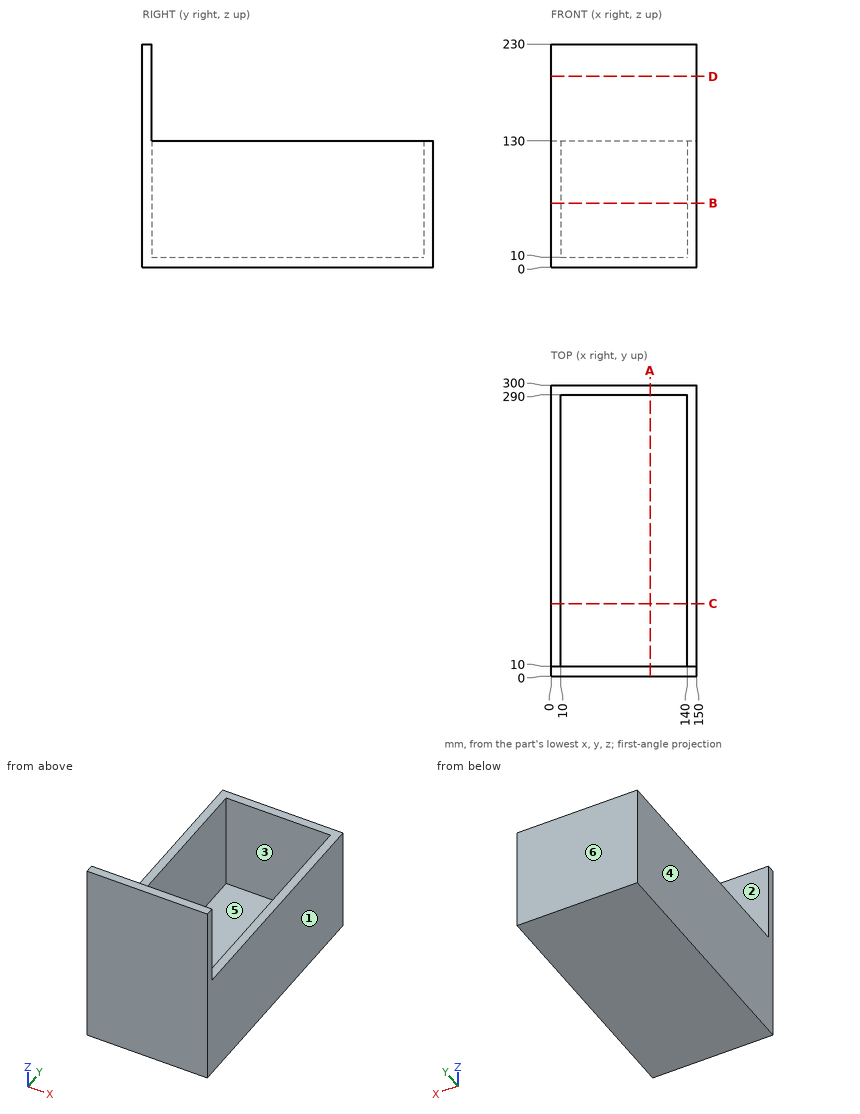
For this review, use the dimensioned drawing (mm, ordinates from the lowest corner) and the shaded views. A direction names the side the tool comes from. Round coordinates to 2 decimals unless told otherwise and drop trailing zeros. Order: outer loops, then holes, each group sorted by start corner. A loop starts at its lowest first (then second) coordinate and runs counter-clockwise, first axis right, second up. Notation, with made-up numbers: M -4,64.5 L 41,64.5 A19 ccw 41,100.5 Z; hole C -10,-33.75 d2. An arc over 180 degrees is marked long. Use a Markdown table: item, result. Add a question column.
Item 1: Tool access review of the marked faces 5 and 6: name each direction out of +Z, -Z, +X, -X, +Y, -Y from which nothing blocks a thin tool from reaching the whole face with its end or side.
Item 2: Mouldability with a two-part tool opening along X and no side actions: class the marked faces 1, 2, 3 and 4 as released by +X, released by -X, zero draft, split by the parting line, or undercut.
Item 3: Add section A-A, the plane x = 102. Give the boundary of the cut face in (y, z), then the cut area to 3 significant figures.
Item 4: Add section B-B, the plane z = 66. Give the boundary of the cut face in (x, y).
Item 5: Add section C-C, the plane y = 74.5. Give the boundary of the cut face in (x, z), then the cut area to 3 significant figures.
Item 6: Insertion check: pin 1 (1.5 mm diameter, centred on x = 57.5, y = 164, fed in from -Z); pin 2 (1 mm diameter, centred on x = 71, z = 185.5, fed in from +Y); pin 3 (4 mm diameter, centred on x = 103, y = 45, fed in from +Z). Each pin has a flat end and moves straight along its axis. Give the tip position at first contact, or say it passes through.
Item 7: To check wall thickness, follow line 1 along Y through (x, z) = (92, 97); line 2 along X through (y, z) = (274.5, 87); line 3 along Y through (x, z) = (89.5, 167.5). State the ranges of each line that lie inside material, in increasing order.
Item 8: Add section D-D, the plane z = 196.5. Give the boundary of the cut face in (x, y), then the cut area to 3 significant figures.
Geometry results:
| question | item | result |
|---|---|---|
| 1 | face 5 | +Z |
| 1 | face 6 | +Z, -Z, +X, -X, +Y |
| 2 | face 1 | released by +X |
| 2 | face 2 | undercut |
| 2 | face 3 | undercut |
| 2 | face 4 | released by -X |
| 3 | outline | M 0,0 L 300,0 L 300,130 L 290,130 L 290,10 L 10,10 L 10,230 L 0,230 Z |
| 3 | area | 6,400 mm² |
| 4 | outline | M 0,0 L 150,0 L 150,300 L 0,300 Z; hole M 10,10 L 140,10 L 140,290 L 10,290 Z |
| 5 | outline | M 0,0 L 150,0 L 150,130 L 140,130 L 140,10 L 10,10 L 10,130 L 0,130 Z |
| 5 | area | 3,900 mm² |
| 6 | pin 1 | stops at z = 0 |
| 6 | pin 2 | stops at y = 10 |
| 6 | pin 3 | stops at z = 10 |
| 7 | line 1 | y = 0 to 10, 290 to 300 |
| 7 | line 2 | x = 0 to 10, 140 to 150 |
| 7 | line 3 | y = 0 to 10 |
| 8 | outline | M 0,0 L 150,0 L 150,10 L 0,10 Z |
| 8 | area | 1,500 mm² |
